Check sheet for the modelled part. Datum: model origin and axes. Units: mm. A direction names the side the tool comes from. Round coordinates to 2 decimals unless told otherwise and drop trailing zeros. Loops run counter-clockwise (first coordinate to the right, second up) from the corner with the lowest first, then second, coordinate; pieces in that order, holes last. Notation, with made-up numbers: (50.5, 80) - (108.5, 80) arc R13 ccw to (108.5, 86) - close; hole circle Ø4 at (63, 63). An arc over 180 degrees is marked (long way). Return JSON: item names as keys, results as strings.
from build123d import *

# Parameters (mm, degrees)
BOSS_EXTRUDE1_DEPTH = 12.5
BOSS_EXTRUDE2_DEPTH = 7.5
BOSS_EXTRUDE3_DEPTH = 7.5
SKETCH5_W           = 70
SKETCH5_H           = 25
CUT_EXTRUDE1_DEPTH  = 10
CUT_EXTRUDE2_START  = -1.632728
SKETCH6_W           = 7.078863834
SKETCH6_H           = 10
CUT_EXTRUDE2_DEPTH  = 1.632728
BOSS_EXTRUDE4_DEPTH = 2
FILLET1_R           = 7
SKETCH8_R           = 2
CUT_EXTRUDE3_DEPTH  = 40
CHAMFER1_SIZE       = 1


with BuildPart() as part:
    # Sketch1 → Boss-Extrude1 (new, symmetric)
    with BuildSketch(Plane.XY):
        with BuildLine():
            Line((22, 2.58125), (22, -7.41875))
            Line((22, -7.41875), (35, -7.41875))
            Line((35, -7.41875), (35, -10.91875))
            Line((35, -10.91875), (22, -10.91875))
            Line((22, -10.91875), (-22, -10.91875))
            Line((-22, -10.91875), (-35, -10.91875))
            Line((-35, -10.91875), (-35, -7.41875))
            Line((-35, -7.41875), (-22, -7.41875))
            Line((-22, -7.41875), (-22, 2.58125))
            Line((-22, 2.58125), (-22, 7.577421516))
            Line((-22, 7.577421516), (-13.039431917, 7.577421516))
            ThreePointArc((-13.039431917, 7.577421516), (0, -9.41875), (13.039431917, 7.577421516))
            Line((13.039431917, 7.577421516), (22, 7.577421516))
            Line((22, 7.577421516), (22, 2.58125))
        make_face()
    extrude(amount=BOSS_EXTRUDE1_DEPTH, both=True)

    # Sketch2 → Boss-Extrude2 (add)
    with BuildSketch(Plane.XY.offset(5)):
        with BuildLine():
            Line((-3.539431917, 5.944693506), (-3.539431917, 7.577421516))
            Line((-3.539431917, 7.577421516), (-13.039431917, 7.577421516))
            ThreePointArc((-13.039431917, 7.577421516), (0, -9.41875), (13.039431917, 7.577421516))
            Line((13.039431917, 7.577421516), (3.539431917, 7.577421516))
            Line((3.539431917, 7.577421516), (3.539431917, 5.944693506))
            ThreePointArc((3.539431917, 5.944693506), (0, 0.08125), (-3.539431917, 5.944693506))
        make_face()
    extrude(amount=BOSS_EXTRUDE2_DEPTH)

    # Sketch3 → Boss-Extrude3 (add)
    with BuildSketch(Plane.XY.offset(-5)):
        with BuildLine():
            Line((3.539431917, 7.577421516), (3.539431917, 5.944693506))
            ThreePointArc((3.539431917, 5.944693506), (0, 0.08125), (-3.539431917, 5.944693506))
            Line((-3.539431917, 5.944693506), (-3.539431917, 7.577421516))
            Line((-3.539431917, 7.577421516), (-13.039431917, 7.577421516))
            ThreePointArc((-13.039431917, 7.577421516), (0, -9.41875), (13.039431917, 7.577421516))
            Line((13.039431917, 7.577421516), (3.539431917, 7.577421516))
        make_face()
    extrude(amount=-BOSS_EXTRUDE3_DEPTH)

    # Sketch4 → Revolve1 (revolve)
    with BuildSketch(Plane(origin=(0, 4.08125, 0), x_dir=(1, 0, 0), z_dir=(0, 1, 0)), mode=Mode.PRIVATE) as revolve1_sk:
        Polygon((-4, -5), (-4, -3.5), (-6, -3.5), (-8.289431917, -5), align=None)
        Polygon((-4, 5), (-4, 3.5), (-6, 3.5), (-8.289431917, 5), align=None)
    revolve(revolve1_sk.sketch.rotate(Axis((0, 4.08125, 0), (0, 0, -1)), 27.765950742), axis=Axis((0, 4.08125, 0), (0, 0, -1)))

    # Sketch5 → Cut-Extrude1 (cut)
    with BuildSketch(Plane(origin=(0, 7.577421516, 0), x_dir=(1, 0, 0), z_dir=(0, 1, 0))):
        Rectangle(SKETCH5_W, SKETCH5_H)
    extrude(amount=CUT_EXTRUDE1_DEPTH, mode=Mode.SUBTRACT)

    # Sketch6 → Cut-Extrude2 (cut)
    with BuildSketch(Plane(origin=(0, 7.577421516, 0), x_dir=(1, 0, 0), z_dir=(0, 1, 0)).offset(CUT_EXTRUDE2_START)):
        Rectangle(SKETCH6_W, SKETCH6_H)
    extrude(amount=CUT_EXTRUDE2_DEPTH, mode=Mode.SUBTRACT)

    # Sketch7 → Boss-Extrude4 (add)
    with BuildSketch(Plane.XY.offset(12.5)):
        Polygon((-22, 2.38125), (-22, 7.577421516), (22, 7.577421516), (22, -3.038829349), (22, -10.91875), (-22, -10.91875), align=None)
    boss_extrude4 = extrude(amount=-BOSS_EXTRUDE4_DEPTH)

    # Mirror1: Boss-Extrude4 across plane
    add(boss_extrude4.mirror(Plane.XY))

    # Fillet1
    fillet1_edges = [part.edges().sort_by_distance(p)[0] for p in [
        (35, -9.16875, -12.5),
        (-35, -9.16875, -12.5),
        (-35, -9.16875, 12.5),
        (35, -9.16875, 12.5),
    ]]
    fillet(fillet1_edges, radius=FILLET1_R)

    # Sketch8 → Cut-Extrude3 (cut)
    with BuildSketch(Plane(origin=(0, -7.41875, 0), x_dir=(1, 0, 0), z_dir=(0, 1, 0))):
        with Locations(Location((28.5, 0, 0), (0, 0, 180))):
            Circle(SKETCH8_R)
        with Locations(Location((-28.5, 0, 0), (0, 0, 180))):
            Circle(SKETCH8_R)
    extrude(amount=-CUT_EXTRUDE3_DEPTH, mode=Mode.SUBTRACT)

    # Chamfer1
    chamfer1_edges = [part.edges().sort_by_distance(p)[0] for p in [
        (0, 7.577421516, -12.5),
        (22, 7.577421516, 0),
        (-22, 7.577421516, 0),
        (0, 7.577421516, 12.5),
    ]]
    chamfer(chamfer1_edges, length=CHAMFER1_SIZE)


solid = part.part
Q1. Sectioned sample at B-B (z = 0.75). Enter the section's corners in (x, y).
Answer key:
{"outline": "(-35, -10.92) - (-30.35, -10.92) - (-30.35, -7.42) - (-35, -7.42) - close; (-26.65, -10.92) - (26.65, -10.92) - (26.65, -7.42) - (22, -7.42) - (22, 6.58) - (21, 7.58) - (13.04, 7.58) arc R13.5 cw (long way) to (-13.04, 7.58) - (-21, 7.58) - (-22, 6.58) - (-22, -7.42) - (-26.65, -7.42) - close; (30.35, -10.92) - (35, -10.92) - (35, -7.42) - (30.35, -7.42) - close"}
Q2. Scan lines: probe 1 along X at (y, z) = (-1, -3.25); probe 2 along Z at (x, y) = (-2.5, 4.5); probe 3 along Z at (x, y) = (8.5, -5). Record each from-to range of solid material in increasing order. Write a range as [from, to].
Answer key:
{"probe 1": "x = [-22, -12.51], [12.51, 22]", "probe 2": "z = [-12.5, -10.5], [10.5, 12.5]", "probe 3": "z = [-12.5, -5], [5, 12.5]"}
Q3. Tool access check on faces 1 (the face through (33, -9.2, 10.4)), 2 (the face through (26, -7.419, 0)), 3 (the face through (-22, -1, 0)), 4 (the face through (0, -5, 5)), 5 (the face through (3.539, 7, 7)). Record the directions out of +Z, -Z, +X, -X, +Y, -Y that give a thin tool (end or side, any length) a straight path to the whole face; none if there is none.
Answer key:
{"face 1": "+Z, +X, +Y, -Y", "face 2": "+Z, -Z, +X, +Y", "face 3": "+Z, -Z, -X, +Y", "face 4": "none", "face 5": "+Y"}
Q4. Sectioned sample at C-C (y = -6.5). Enter the section's corners in (x, z), plus the area to 3 significant figures.
Answer key:
{"outline": "(-22, -12.5) - (22, -12.5) - (22, 12.5) - (-22, 12.5) - close; hole (-8.38, -5) - (8.38, -5) - (8.38, 5) - (-8.38, 5) - close", "area": "932 mm²"}
Q5. Draft check along Y on faces 6 (the face through (0, -10.919, 0)), 7 (the face through (0.189, -2.059, -3.594)), 8 (the face through (-30.408, -9.144, 0.601)), 9 (the face through (-0.346, -9.414, 0.07)). Enter one of: released by +Y, released by -Y, zero draft, split by the parting line, or undercut.
Answer key:
{"face 6": "released by -Y", "face 7": "undercut", "face 8": "zero draft", "face 9": "undercut"}
Q6. Depth check by flat-ended pin: P1, Ø1.3, axis at y = 7, z = 7, coming from the -X side; P2, Ø5, axis at y = -3, z = -2, coming from the +X side; P3, Ø5, axis at x = 28.5, z = 0, coming from the +Y side. Enter the tip coordinate at first touch or a pass-through.
Answer key:
{"P1": "stops at x = -22", "P2": "stops at x = 22", "P3": "stops at y = -7.42"}
Q7. Sectioned sample at D-D (z = -7.25). Enter the section's corners in (x, y), plus the area to 3 significant figures.
Answer key:
{"outline": "(-34.78, -10.92) - (34.78, -10.92) - (34.78, -7.42) - (22, -7.42) - (22, 6.58) - (21, 7.58) - (3.54, 7.58) - (3.54, 5.94) arc R4 cw (long way) to (-3.54, 5.94) - (-3.54, 7.58) - (-21, 7.58) - (-22, 6.58) - (-22, -7.42) - (-34.78, -7.42) - close", "area": "851 mm²"}
Q8. Sectioned sample at A-A (x = 0). Enter the section's corners in (y, z).
Answer key:
{"outline": "(-10.92, -12.5) - (6.58, -12.5) - (7.58, -11.5) - (7.58, -10.5) - (0.08, -10.5) - (0.08, -3.5) - (-1.92, -3.5) - (-4.21, -5) - (-9.42, -5) - (-9.42, 5) - (-4.21, 5) - (-1.92, 3.5) - (0.08, 3.5) - (0.08, 10.5) - (7.58, 10.5) - (7.58, 11.5) - (6.58, 12.5) - (-10.92, 12.5) - close"}
